Work out the finished part from the listing and answer in its coordinate system (mm). Face numbers are marked on the shaded views. Coordinates: 2 decimals unless noted, no trailing zeros. Loops run counter-clockwise (first coordinate to the right, second up) from the corner with the lowest first, then second, coordinate; pieces in that order, holes last. Notation, with made-up numbers: (78, -30.5) -> (117, -30.5) arc R21 cw to (117, -16.5) -> close; hole circle Ø4 at (61, 20). An arc over 180 degrees is marked (long way). Answer as CSV lines item,"result".
```python
from build123d import *

# Parameters (mm, degrees)
F1_DEPTH = 101.6
F2_R     = 5.08


with BuildPart() as f1:
    # F0 (on Right) → F1 (new body, symmetric)
    with BuildSketch(Plane.YZ):
        Polygon((52.1238698428, 143.2091554078), (0, 0), (63.5, 0), (63.5, 6.3499992049), (9.0687387073, 6.3499992049), (58.8813978519, 143.2091554078), align=None)
    extrude(amount=F1_DEPTH, both=True)

    # F2
    f2_edges = [f1.edges().sort_by_distance(p)[0] for p in [
        (0, 0, 0),
    ]]
    fillet(f2_edges, radius=F2_R)


solid = f1.part
```
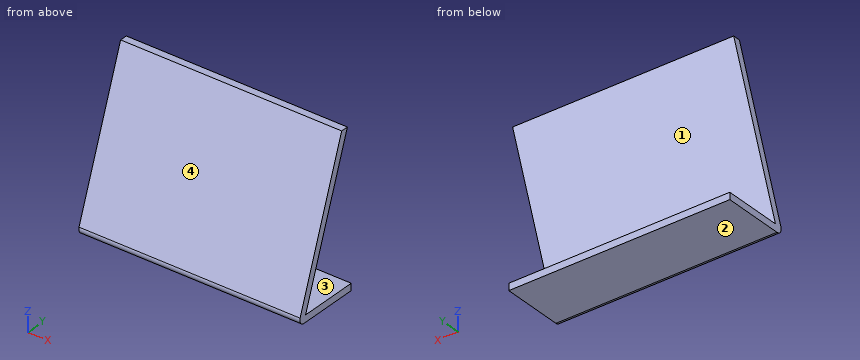
(1) Consider line 1 along Y through (x, z) = (-16, 91.5); line 2 along Y through (x, z) = (38, 67.5). Determine where each line is inside the solid, lowest interval first.
Computed values:
line 1,"33.3 to 40.06"
line 2,"24.57 to 31.33"
(2) A cutting plane is placed at C-C, the plane y = 54.5. Write down the section's boundary in (x, z), and give its area (3 significant figures).
Computed values:
outline,"(-101.6, 0) -> (101.6, 0) -> (101.6, 6.35) -> (-101.6, 6.35) -> close; (-101.6, 131.17) -> (101.6, 131.17) -> (101.6, 143.21) -> (-101.6, 143.21) -> close"
area,"3,740 mm2"
(3) A cutting plane is placed at D-D, the plane z = 133.5. Write down the section's boundary in (x, y), and give its area (3 significant figures).
Computed values:
outline,"(-101.6, 48.59) -> (101.6, 48.59) -> (101.6, 55.35) -> (-101.6, 55.35) -> close"
area,"1,370 mm2"
(4) Flat-ended cylindrical pins translate along their axes: pin 1 Ø1 at (x, z) = (49, 77.5) entering from +Y; pin 2 Ø12 at (x, z) = (74, 60.5) entering from -Y; pin 3 Ø2 at (x, z) = (66, 92.5) entering from -Y; pin 4 Ø8 at (y, z) = (25, 44.5) entering from -X. Find the tip coordinate at first contact, or state that the pin passes through.
Computed values:
pin 1,"y = 35.15"
pin 2,"y = 19.84"
pin 3,"y = 33.3"
pin 4,"x = -101.6"
(5) A cutting plane is placed at A-A, the plane y = 27.5. Write down the section's boundary in (x, z).
Computed values:
outline,"(-101.6, 0) -> (101.6, 0) -> (101.6, 6.35) -> (-101.6, 6.35) -> close; (-101.6, 56.99) -> (101.6, 56.99) -> (101.6, 75.56) -> (-101.6, 75.56) -> close"
(6) A cutting plane is placed at B-B, the plane x = 79. Write down the section's boundary in (y, z) (3 decimals), and give its area (3 significant figures).
Computed values:
outline,"(2.481, 6.817) arc R5.08 ccw to (7.255, 0) -> (63.5, 0) -> (63.5, 6.35) -> (9.069, 6.35) -> (58.881, 143.209) -> (52.124, 143.209) -> close"
area,"1,310 mm2"
(7) For a pull along Z with two mould halves and no side action, classify the marked faces 1, 2, 3 and 4 as pulls with the +Z half, pulls with the -Z half, needs draft (parallel to the pull), parting line crosses it, or undercut.
Computed values:
face 1,"undercut"
face 2,"pulls with the -Z half"
face 3,"undercut"
face 4,"pulls with the +Z half"
